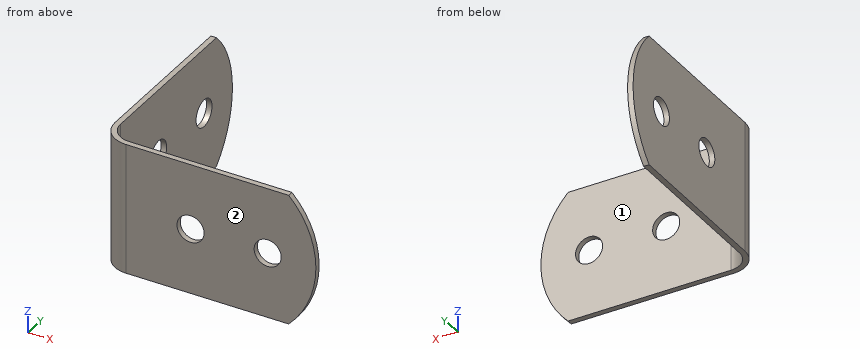
```python
from build123d import *

# Parameters (mm, degrees)
BOSS_EXTRUDE1_DEPTH   = 24.13
FILLET1_R             = 3.81
FILLET2_R             = 4.826
F_5_0MM_DOWEL_HOLE1_D = 5
F_5_0MM_DOWEL_HOLE2_D = 5
CUT_EXTRUDE1_DEPTH    = 40.878
CUT_EXTRUDE2_DEPTH    = 40.878


with BuildPart() as part:
    # Sketch1 → Boss-Extrude1 (new body)
    with BuildSketch(Plane.XY):
        Polygon((0, 39.878), (0, 0), (39.878, 0), (39.878, 1.016), (1.016, 1.016), (1.016, 39.878), align=None)
    extrude(amount=BOSS_EXTRUDE1_DEPTH)

    # Fillet1
    fillet1_edges = [part.edges().sort_by_distance(p)[0] for p in [
        (1.016, 1.016, 12.065),
    ]]
    fillet(fillet1_edges, radius=FILLET1_R)

    # Fillet2
    fillet2_edges = [part.edges().sort_by_distance(p)[0] for p in [
        (0, 0, 12.065),
    ]]
    fillet(fillet2_edges, radius=FILLET2_R)

    # Ø5.0mm Dowel Hole1 (through all)
    with Locations(Plane.ZY):
        with Locations((12.065, 30.988), (12.065, 16.764)):
            Hole(F_5_0MM_DOWEL_HOLE1_D / 2)

    # Ø5.0mm Dowel Hole2 (through all)
    with Locations(Plane(origin=(0, 0, 0), x_dir=(-1, 0, 0), z_dir=(0, -1, 0))):
        with Locations((-30.988, -12.065), (-16.764, -12.065)):
            Hole(F_5_0MM_DOWEL_HOLE2_D / 2)

    # Sketch6 → Cut-Extrude1 (cut, through all)
    with BuildSketch(Plane.XZ):
        with BuildLine():
            Line((34.862003958, 24.13), (44.45, 24.13))
            Line((44.45, 24.13), (44.45, 0))
            Line((44.45, 0), (34.862003958, 0))
            ThreePointArc((34.862003958, 0), (39.878, 12.065), (34.862003958, 24.13))
        make_face()
    extrude(amount=-CUT_EXTRUDE1_DEPTH, mode=Mode.SUBTRACT)

    # Sketch7 → Cut-Extrude2 (cut, through all)
    with BuildSketch(Plane.ZY):
        with BuildLine():
            Line((0, 34.862003958), (0, 44.45))
            Line((0, 44.45), (24.13, 44.45))
            Line((24.13, 44.45), (24.13, 34.862003958))
            ThreePointArc((24.13, 34.862003958), (12.065, 39.878), (0, 34.862003958))
        make_face()
    extrude(amount=-CUT_EXTRUDE2_DEPTH, mode=Mode.SUBTRACT)


solid = part.part
```
Geometry check sheet. Reference: the model listing, model coordinates, mm. Face numbers are marked on the shaded views. A direction names the side the tool comes from. Give positions to 0.01 mm unless a question says otherwise; leave off trailing zeros. Write each loop counter-clockwise with the first axis right and the second up, starting at its lowest first coordinate (ties: lowest second). Pieces come first, ordered by that corner, then holes.
1) Section check B-B, the plane z = 11.5. Record the boundary of the cut face in (x, y), and give its area (3 significant figures).
2) Section check A-A, the plane x = 15. Record the boundary of the cut face in (y, z), and give its area (3 significant figures).
3) Section check D-D, the plane z = 4. Record the boundary of the cut face in (x, y), and give its area (3 significant figures).
4) Access from +Z, -Z, +X, -X, +Y, -Y to the whole of each face (thin tool, end or side, straight path). Record for the marked faces 1 and 2.
5) Gauge pin test, flat ends, axial feed: pin 1 (8 mm diameter, centred on x = 30.988, z = 12.065, fed in from +Y); pin 2 (4 mm diameter, centred on y = 16, z = 11, fed in from +X). Record the tip position at first contact, or that the pin passes through.
6) Section check C-C, the plane y = 29.5. Record the boundary of the cut face in (x, z).
7) Material ranges on L1, parallel to Y at x = 18, z = 22; L2, parallel to X at y = 3, z = 6.5, recorded low to high.
Computed:
1. outline: (0, 4.83) arc R4.83 ccw to (4.83, 0) - (14.33, 0) - (14.33, 1.02) - (4.83, 1.02) arc R3.81 cw to (1.02, 4.83) - (1.02, 14.33) - (0, 14.33) - close; (0, 19.2) - (1.02, 19.2) - (1.02, 28.55) - (0, 28.55) - close; (0, 33.42) - (1.02, 33.42) - (1.02, 39.87) - (0, 39.87) - close; (19.2, 0) - (28.55, 0) - (28.55, 1.02) - (19.2, 1.02) - close; (33.42, 0) - (39.87, 0) - (39.87, 1.02) - (33.42, 1.02) - close
1. area: 58.3 mm2
2. outline: (0, 0) - (1.02, 0) - (1.02, 10.29) - (0, 10.29) - close; (0, 13.84) - (1.02, 13.84) - (1.02, 24.13) - (0, 24.13) - close
2. area: 20.9 mm2
3. outline: (0, 4.83) arc R4.83 ccw to (4.83, 0) - (37.85, 0) - (37.85, 1.02) - (4.83, 1.02) arc R3.81 cw to (1.02, 4.83) - (1.02, 37.85) - (0, 37.85) - close
3. area: 74.0 mm2
4. face 1: +Z, -Z, +X, +Y
4. face 2: +Z, -Z, +X, -X, -Y
5. pin 1: stops at y = 1.02
5. pin 2: stops at x = 1.02
6. outline: (0, 0) - (1.02, 0) - (1.02, 10.06) - (0, 10.06) - close; (0, 14.07) - (1.02, 14.07) - (1.02, 24.13) - (0, 24.13) - close
7. L1: y = 0 to 1.02
7. L2: x = 0.36 to 1.48
